Answer from the drawing. Dimensions are ordinates in mm from the lowest x, y and z of the part. Coordinates: 2 decimals unless noted, no trailing zeros. Write each loop counter-clockwise with the first axis right and the second up, starting at its lowest first coordinate (ties: lowest second). Pieces come first, ordered by that corner, then holes. Notation, with made-up numbers: (12.5, 87) -> (56.5, 87) arc R24 cw to (56.5, 116) -> close; hole circle Ø6 at (35, 63). An arc over 180 degrees is marked (long way). Answer as a JSON object with one key per item and string values. Group by question number.
(1) A flat-ended cylindrical pin translates along its axis: P1, Ø21.5, axis at y = 297.5, z = 82, coming from the +X side. Find the tip coordinate at first contact, or state that the pin passes through.
(2) Find section A-A (z = 82). Give the vertices of the cut face in (x, y), then the cut area to 3 significant figures.
(3) Find section C-C (y = 147.5). Give the vertices of the cut face in (x, z), then the cut area to 3 significant figures.
(4) Find section D-D (y = 301). Give the vertices of the cut face in (x, z), then the cut area to 3 significant figures.
(5) Straight lines are drawn through the part: L1, parallel to Z at x = 7.75, y = 297.5; L2, parallel to Y at x = 5.5, z = 93; L3, parallel to Y at x = 8.75, z = 87. For each, find the intervals that lie inside material, in ascending order.
(6) Find section B-B (x = 6.25). Give the vertices of the cut face in (y, z), then the cut area to 3 significant figures.
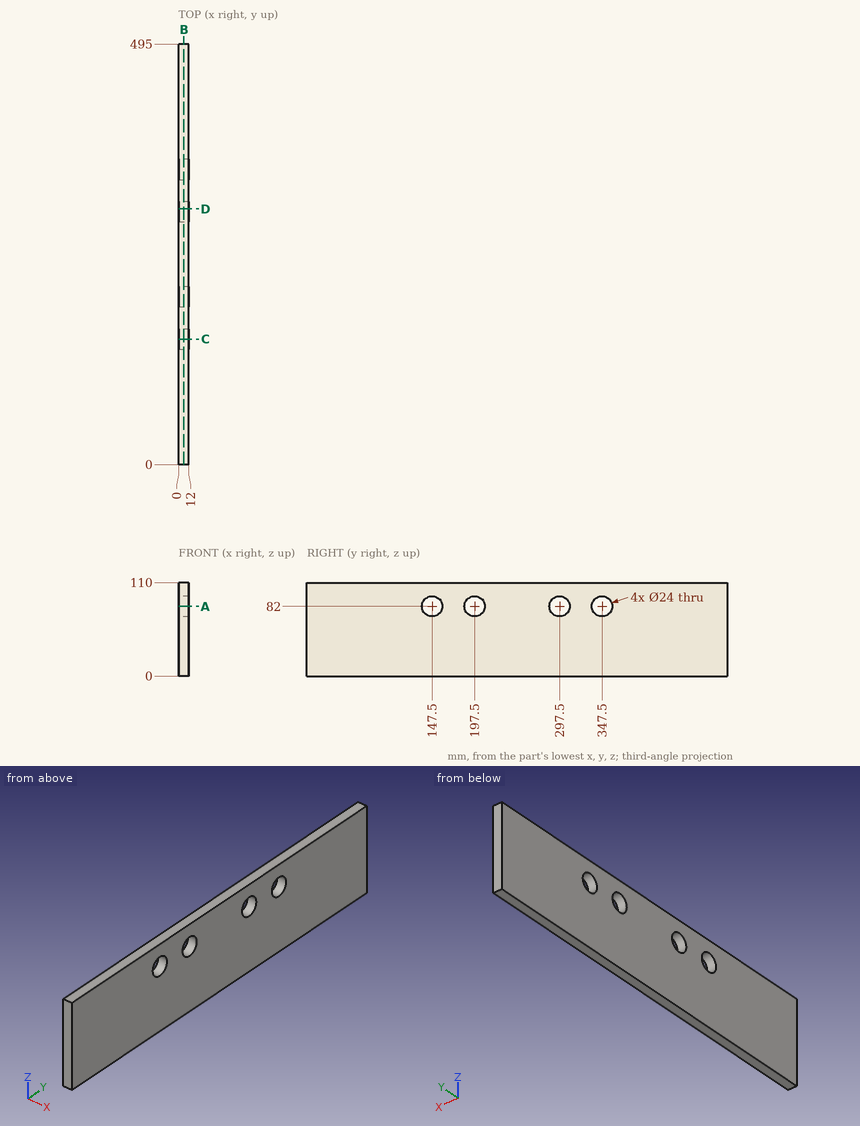
Results below:
{
 "1": {"P1": "passes through"},
 "2": {"outline": "(0, 0) -> (12, 0) -> (12, 135.5) -> (0, 135.5) -> close; (0, 159.5) -> (12, 159.5) -> (12, 185.5) -> (0, 185.5) -> close; (0, 209.5) -> (12, 209.5) -> (12, 285.5) -> (0, 285.5) -> close; (0, 309.5) -> (12, 309.5) -> (12, 335.5) -> (0, 335.5) -> close; (0, 359.5) -> (12, 359.5) -> (12, 495) -> (0, 495) -> close", "area": "4,790 mm2"},
 "3": {"outline": "(0, 0) -> (12, 0) -> (12, 70) -> (0, 70) -> close; (0, 94) -> (12, 94) -> (12, 110) -> (0, 110) -> close", "area": "1,030 mm2"},
 "4": {"outline": "(0, 0) -> (12, 0) -> (12, 70.52) -> (0, 70.52) -> close; (0, 93.48) -> (12, 93.48) -> (12, 110) -> (0, 110) -> close", "area": "1,040 mm2"},
 "5": {"L1": "z = 0 to 70, 94 to 110", "L2": "y = 0 to 142.7, 152.3 to 192.7, 202.3 to 292.7, 302.3 to 342.7, 352.3 to 495", "L3": "y = 0 to 136.59, 158.41 to 186.59, 208.41 to 286.59, 308.41 to 336.59, 358.41 to 495"},
 "6": {"outline": "(0, 0) -> (495, 0) -> (495, 110) -> (0, 110) -> close; hole circle Ø24 at (147.5, 82); hole circle Ø24 at (197.5, 82); hole circle Ø24 at (297.5, 82); hole circle Ø24 at (347.5, 82)", "area": "52,600 mm2"}
}
